The model under review builds one solid part; all positions refer to its coordinate system, in mm. A direction names the side the tool comes from. Coordinates: 2 decimals unless noted, no trailing zeros. Write each loop counter-clockwise with the first axis right and the second up, starting at its lowest first coordinate (ties: lowest second). Pieces come first, ordered by that corner, then holes.
Autodesk Inventor part; units mm, degrees
ref_plane "YZ Plane" through (0, 0, 0) normal (1, 0, 0) x (0, 1, 0)
ref_plane "XZ Plane" through (0, 0, 0) normal (0, 1, 0) x (-1, 0, 0)
ref_plane "XY Plane" through (0, 0, 0) normal (0, 0, 1) x (1, 0, 0)
sketch "Sketch1" plane through (0, 0, 0) normal (0, 0, 1) x (1, 0, 0)
  line L0 (-15.5, 15.5) -> (15.5, 15.5)
  line L1 (15.5, 15.5) -> (15.5, -15.5)
  line L2 (15.5, -15.5) -> (-15.5, -15.5)
  line L3 (-15.5, -15.5) -> (-15.5, 15.5)
  line L4 (29.5, 15.5) -> (60.5, 15.5)
  line L5 (60.5, 15.5) -> (60.5, -15.5)
  line L6 (60.5, -15.5) -> (29.5, -15.5)
  line L7 (29.5, -15.5) -> (29.5, 15.5)
  line L8 (-20.5, 20.5) -> (65.5, 20.5)
  line L9 (65.5, 20.5) -> (65.5, -20.5)
  line L10 (65.5, -20.5) -> (-20.5, -20.5)
  line L11 (-20.5, -20.5) -> (-20.5, 20.5)
  circle A0 centre (0, 0) radius 11
  circle A1 centre (45, 0) radius 11
  dimension "d0" = 31
  dimension "d5" = 45
  dimension "d10" = 5
  dimension "d11" = 5
  dimension "d12" = 5
  dimension "d13" = 5
  dimension "d16" = 22
extrude "Extrusion1" add sketch "Sketch1" along normal blind 8 contours L0 L1 L2 L3 | L4 L5 L6 L7 | L8 L9 L10 L11 | A0 | A1
sketch "Sketch2" plane through (0, 0, 0) normal (0, 0, 1) x (1, 0, 0)
  circle A0 centre (45, 0) radius 11
  point P0 (0, 0)
sketch "Sketch4" plane through (0, 0, 8) normal (0, 0, 1) x (1, 0, 0)
  point P0 (0, 0)
  point P1 (15.5, 15.5)
  point P2 (-15.5, 15.5)
  point P3 (-15.5, -15.5)
  point P4 (15.5, -15.5)
hole "Hole3" at (-15.5, 15.5, 8) at (15.5, 15.5, 8) at (15.5, -15.5, 8) at (-15.5, -15.5, 8) direction (0, 0, -1) diameter 3.2 end through all countersink diameter 6.3 countersink angle 90
sketch "Sketch16" plane through (0, 0, 0) normal (0, 0, 1) x (1, 0, 0)
  line L0 (65.5, 20.5) -> (-20.5, 20.5)
  line L1 (-20.5, -20.5) -> (65.5, -20.5)
  line L2 (24.5, 20.5) -> (65.5, 20.5)
  line L3 (65.5, 20.5) -> (65.5, -20.5)
  line L4 (65.5, -20.5) -> (24.5, -20.5)
  line L5 (24.5, -20.5) -> (24.5, 20.5)
  point P0 (0, 0)
extrude "Extrusion7" add sketch "Sketch16" against normal blind 10
sketch "Sketch18" plane through (0, 0, 8) normal (0, 0, 1) x (1, 0, 0)
  line L0 (29.5, 15.5) -> (60.5, 15.5)
  line L1 (29.5, -15.5) -> (29.5, 15.5)
  line L2 (60.5, -15.5) -> (29.5, -15.5)
  line L3 (60.5, 15.5) -> (60.5, -15.5)
  point P0 (0, 0)
sketch "Sketch14" plane through (0, 0, 8) normal (0, 0, -1) x (-1, 0, 0)
  circle A0 centre (-45, 0) radius 11
  point P0 (0, 0)
  point P1 (-46.783, 15.548)
  dimension "d178" = 1.783
  dimension "d179" = 15.548
hole "Hole5" at (46.783, 15.548, 8) direction (0, 0, -1) diameter 6.5 end through all
sketch "Sketch13" plane through (0, 0, 8) normal (0, 0, -1) x (-1, 0, 0)
  line L0 (-62.0877, 18.25) -> (-58.9123, 18.25)
  line L1 (-58.9123, 18.25) -> (-57.3246, 15.5)
  line L2 (-57.3246, 15.5) -> (-58.9123, 12.75)
  line L3 (-58.9123, 12.75) -> (-62.0877, 12.75)
  line L4 (-62.0877, 12.75) -> (-63.6754, 15.5)
  line L5 (-63.6754, 15.5) -> (-62.0877, 18.25)
  line L6 (-31.0877, 18.25) -> (-27.9123, 18.25)
  line L7 (-27.9123, 18.25) -> (-26.3246, 15.5)
  line L8 (-26.3246, 15.5) -> (-27.9123, 12.75)
  line L9 (-27.9123, 12.75) -> (-31.0877, 12.75)
  line L10 (-31.0877, 12.75) -> (-32.6754, 15.5)
  line L11 (-32.6754, 15.5) -> (-31.0877, 18.25)
  line L12 (-62.0877, -12.75) -> (-58.9123, -12.75)
  line L13 (-58.9123, -12.75) -> (-57.3246, -15.5)
  line L14 (-57.3246, -15.5) -> (-58.9123, -18.25)
  line L15 (-58.9123, -18.25) -> (-62.0877, -18.25)
  line L16 (-62.0877, -18.25) -> (-63.6754, -15.5)
  line L17 (-63.6754, -15.5) -> (-62.0877, -12.75)
  line L18 (-31.0877, -12.75) -> (-27.9123, -12.75)
  line L19 (-27.9123, -12.75) -> (-26.3246, -15.5)
  line L20 (-26.3246, -15.5) -> (-27.9123, -18.25)
  line L21 (-27.9123, -18.25) -> (-31.0877, -18.25)
  line L22 (-31.0877, -18.25) -> (-32.6754, -15.5)
  line L23 (-32.6754, -15.5) -> (-31.0877, -12.75)
  point P0 (0, 0)
  point P1 (-60.5, 15.5)
  point P2 (-29.5, 15.5)
  point P3 (-60.5, -15.5)
  point P4 (-29.5, -15.5)
  point P5 (-60.5, 15.5)
  point P6 (-29.5, 15.5)
  point P7 (-60.5, -15.5)
  point P8 (-29.5, -15.5)
  point P9 (-45, 0)
  dimension "d129" = 5.5
extrude "Extrusion6" cut sketch "Sketch13" along normal blind 3.6
hole "Hole7" at (45, 0, 8) direction (0, 0, -1) diameter 8 end through all counterbore diameter 22 counterbore depth 7
hole "Hole8" at (29.5, 15.5, 8) at (60.5, 15.5, 8) at (60.5, -15.5, 8) at (29.5, -15.5, 8) direction (0, 0, -1) diameter 3.2 end through all
hole "Hole9" at (0, 0, 0) direction (0, 0, 1) diameter 6 end through all counterbore diameter 23 counterbore depth 2.2
equation "\"d64\" = 55deg"
equation "\"Sketch5_Pitch\" = 0.5"
equation "\"d82\" = 55deg"
equation "\"Sketch7_Pitch\" = 0.5"
equation "\"d100\" = 55deg"
equation "\"Sketch9_Pitch\" = 0.5"
equation "\"d118\" = 55deg"
equation "\"Sketch11_Pitch\" = 0.5"
properties part number "ReductionGearBracket"
Item 1: Machinability: for faces 3 (the face through (-11.4, -1.5, 1.1)), 4 (the face through (22, 0, 8)), 5 (the face through (59, -17, 4.4)), which of the approach directions +Z, -Z, +X, -X, +Y, -Y give a long, thin tool a straight path to every point of the face, cutting with its end or side? Answer none if there is none.
Solved:
face 3: -Z
face 4: +Z, +X, -X, +Y, -Y
face 5: +Z
Item 2: Take a section at B-B, the plane y = 0. Write out the cut boundary in (x, z).
Solved:
outline: (-20.5, 0) - (-11.5, 0) - (-11.5, 2.2) - (-3, 2.2) - (-3, 8) - (-20.5, 8) - close; (3, 2.2) - (11.5, 2.2) - (11.5, 0) - (24.5, 0) - (24.5, -10) - (41, -10) - (41, 1) - (34, 1) - (34, 8) - (3, 8) - close; (49, -10) - (65.5, -10) - (65.5, 8) - (56, 8) - (56, 1) - (49, 1) - close
Item 3: Mouldability with a two-part tool opening along Y and no side actions: class faces 1 (the face through (31.89, 16.86, 6.23)), 2 (the face through (24.5, 0, -5)) as pulls with the +Y half, pulls with the -Y half, needs draft (parallel to the pull), parting line crosses it, or undercut.
Solved:
face 1: undercut
face 2: needs draft
Item 4: To check wall thickness, follow line 1 along X through (y, z) = (15.5, -6); line 2 along X through (y, z) = (0, 0.9); line 3 along Y through (x, z) = (60.5, 1). State the ranges of each line that lie inside material, in increasing order.
Solved:
line 1: x = 24.5 to 27.9, 31.1 to 43.53, 50.03 to 58.9, 62.1 to 65.5
line 2: x = -20.5 to -11.5, 11.5 to 41, 49 to 65.5
line 3: y = -20.5 to -17.1, -13.9 to 13.9, 17.1 to 20.5
Item 5: Take a section at A-A, the plane x = -15.5. Write out the cut boundary in (y, z).
Solved:
outline: (-20.5, 0) - (-17.1, 0) - (-17.1, 6.45) - (-18.65, 8) - (-20.5, 8) - close; (-13.9, 0) - (13.9, 0) - (13.9, 6.45) - (12.35, 8) - (-12.35, 8) - (-13.9, 6.45) - close; (17.1, 0) - (20.5, 0) - (20.5, 8) - (18.65, 8) - (17.1, 6.45) - close
Item 6: Take a section at C-C, the plane x = 0. Write out the cut boundary in (y, z), plus the area to 3 significant figures.
Solved:
outline: (-20.5, 0) - (-11.5, 0) - (-11.5, 2.2) - (-3, 2.2) - (-3, 8) - (-20.5, 8) - close; (3, 2.2) - (11.5, 2.2) - (11.5, 0) - (20.5, 0) - (20.5, 8) - (3, 8) - close
area: 243 mm2
Item 7: For pin 1 (3.5 mm diameter, centred on x = 60.5, y = -15.5, fed in from +Z); pin 2 (3 mm diameter, centred on y = -9.5, z = -7, fed in from -X); pin 3 (11 mm diameter, centred on x = 44, y = 4, fed in from +Z), all flat-tipped, find the tip position at first contact; note any pin that passes through.
Solved:
pin 1: stops at z = 4.4
pin 2: stops at x = 24.5
pin 3: stops at z = 1
Item 8: Take a section at D-D, the plane z = -7.25. Write out the cut boundary in (x, y).
Solved:
outline: (24.5, -20.5) - (65.5, -20.5) - (65.5, 20.5) - (24.5, 20.5) - close; hole circle Ø3.2 at (29.5, -15.5); hole circle Ø3.2 at (29.5, 15.5); hole circle Ø8 at (45, 0); hole circle Ø6.5 at (46.78, 15.55); hole circle Ø3.2 at (60.5, -15.5); hole circle Ø3.2 at (60.5, 15.5)
